The listing builds one solid part. Answer for the finished solid, in the listing's coordinates (mm). A direction names the side the tool comes from. Give positions to 0.01 mm unless a question says otherwise; leave off trailing zeros. Order: outer loops, then holes, each group sorted by start corner. A loop starts at its lowest first (then second) coordinate and runs counter-clockwise, first axis right, second up. Notation, with made-up numbers: (-32, 82) -> (-5, 82) arc R17 ccw to (-5, 112) -> close; hole circle Ø9 at (-19, -25.5). An arc over 180 degrees is marked (long way). Answer as a JSON object with one key per item and string values. Group by question number.
```python
from build123d import *

# Parameters (mm, degrees)
F0_W     = 115
F0_H     = 53
F0_W_2   = 98
F0_H_2   = 36
F1_DEPTH = 4
F2_W     = 130
F2_H     = 60
F3_DEPTH = 2
F4_DEPTH = 2.001
F5_D     = 3.3
F5_DEPTH = 4.001
F6_W     = 4.3469965458
F6_H     = 25.2998827054
F6_W_2   = 4.7431737185
F6_H_2   = 24.9695125967
F7_DEPTH = 25


with BuildPart() as f1:
    # F0 (on Top) → F1 (new body)
    with BuildSketch(Plane.XY):
        with Locations((-9.9708801619, 5.0761482663)):
            Rectangle(F0_W, F0_H)
        with Locations((-9.9708801619, 5.0761482663)):
            Rectangle(F0_W_2, F0_H_2, mode=Mode.SUBTRACT)
    extrude(amount=F1_DEPTH)

    # F2 (on Top) → F3 (join)
    with BuildSketch(Plane.XY):
        with Locations((-7.2538307309, 5.1540893316)):
            Rectangle(F2_W, F2_H)
    extrude(amount=-F3_DEPTH)

    # F0 (on Top) → F4 (cut, through all)
    with BuildSketch(Plane.XY):
        with Locations((-9.9708801619, 5.0761482663)):
            Rectangle(F0_W_2, F0_H_2)
    extrude(amount=-F4_DEPTH, mode=Mode.SUBTRACT)

    # F5 (through all, one way)
    with BuildSketch(Plane(origin=(0, 0, 0), x_dir=(1, 0, 0), z_dir=(0, 0, -1))):
        with Locations((-56.9708801619, -27.0761482663), (-56.9708801619, 16.9238517337), (37.0291198381, 16.9238517337), (37.0291198381, -27.0761482663)):
            Circle(F5_D / 2)
    extrude(amount=-F5_DEPTH, mode=Mode.SUBTRACT)

    # F6 (on Top) → F7 (join)
    with BuildSketch(Plane.XY):
        with Locations((55.7790957391, -12.1861611478)):
            Rectangle(F6_W, F6_H)
        with Locations((-69.787338376, -12.4847562984)):
            Rectangle(F6_W_2, F6_H_2)
    extrude(amount=F7_DEPTH)


solid = f1.part
```
(1) A cutting plane is placed at C-C (z = 10). Determine the outline of the cut face in (x, y), and give its area (3 significant figures).
(2) A cutting plane is placed at A-A (x = 3.5). Determine the outline of the cut face in (y, z).
(3) For a pull along Y with two mould halves and no side action, classify faces 1 (the flat face through (53.606, -12, 12)), 2 (the flat face through (37, 27, 0)), 3 (the flat face through (-11, 23.076, 1)), 4 (the flat face through (-11, -21.424, 2)) as +Y half, -Y half, draft (parallel to the pull), parting line (faces both ways), or undercut.
(4) Flat-ended cylindrical pins translate along their axes: pin 1 Ø7.5 at (y, z) = (-15.5, 17.5) entering from -X; pin 2 Ø8 at (x, z) = (2.5, 3) entering from -Y; pin 3 Ø4 at (x, z) = (-71, 16) entering from +Y; pin 4 Ø3 at (y, z) = (19.5, 7) entering from +X. Find the tip coordinate at first contact, or state that the pin passes through.
(5) A cutting plane is placed at D-D (z = 1.75). Determine the outline of the cut face in (x, y), and give its area (3 significant figures).
(6) A cutting plane is placed at B-B (y = -5). Determine the outline of the cut face in (x, z).
(7) Find the intervals of material crossed by line 1 along Y through (x, z) = (-21, -0.25); line 2 along X through (y, z) = (-11.5, 10.25); line 3 along X through (y, z) = (16.5, 1.75), in increasing order. Write a range as [from, to].
(8) Which of the six approach directions +Z, -Z, +X, -X, +Y, -Y give full straight-line access (tool end or side, diameter ignored) to faces 5 (the flat face through (-11, -12.924, 1)), 6 (the flat face through (37, -17, 0)), 7 (the flat face through (56, -24.836, 12)), 8 (the flat face through (-72.159, -13, 12))?
Check sheet entries:
{
 "1": {"outline": "(-72.16, -24.97) -> (-67.42, -24.97) -> (-67.42, 0) -> (-72.16, 0) -> close; (53.61, -24.84) -> (57.95, -24.84) -> (57.95, 0.46) -> (53.61, 0.46) -> close", "area": "228 mm2"},
 "2": {"outline": "(-24.85, -2) -> (-12.92, -2) -> (-12.92, 4) -> (-21.42, 4) -> (-21.42, 0) -> (-24.85, 0) -> close; (23.08, -2) -> (35.15, -2) -> (35.15, 0) -> (31.58, 0) -> (31.58, 4) -> (23.08, 4) -> close"},
 "3": {"face 1": "draft", "face 2": "undercut", "face 3": "undercut", "face 4": "-Y half"},
 "4": {"pin 1": "stops at x = -72.16", "pin 2": "stops at y = -24.85", "pin 3": "stops at y = 0", "pin 4": "passes through"},
 "5": {"outline": "(-72.16, -24.97) -> (-67.42, -24.97) -> (-67.42, -21.42) -> (47.53, -21.42) -> (47.53, 31.58) -> (-67.47, 31.58) -> (-67.47, 0) -> (-72.16, 0) -> close; (53.61, -24.84) -> (57.95, -24.84) -> (57.95, 0.46) -> (53.61, 0.46) -> close; hole (-58.97, -12.92) -> (39.03, -12.92) -> (39.03, 23.08) -> (-58.97, 23.08) -> close; hole circle Ø3.3 at (-56.97, -16.92); hole circle Ø3.3 at (-56.97, 27.08); hole circle Ø3.3 at (37.03, -16.92); hole circle Ø3.3 at (37.03, 27.08)", "area": "2,760 mm2"},
 "6": {"outline": "(-72.25, -2) -> (-58.97, -2) -> (-58.97, 4) -> (-67.42, 4) -> (-67.42, 25) -> (-72.16, 25) -> (-72.16, 0) -> (-72.25, 0) -> close; (39.03, -2) -> (57.75, -2) -> (57.75, 0) -> (57.95, 0) -> (57.95, 25) -> (53.61, 25) -> (53.61, 0) -> (47.53, 0) -> (47.53, 4) -> (39.03, 4) -> close"},
 "7": {"line 1": "y = [-24.85, -12.92], [23.08, 35.15]", "line 2": "x = [-72.16, -67.42], [53.61, 57.95]", "line 3": "x = [-67.47, -58.97], [39.03, 47.53]"},
 "8": {"face 5": "+Z, -Z", "face 6": "+Z", "face 7": "+Z, -Z, +X, -Y", "face 8": "+Z, -X, +Y, -Y"}
}
